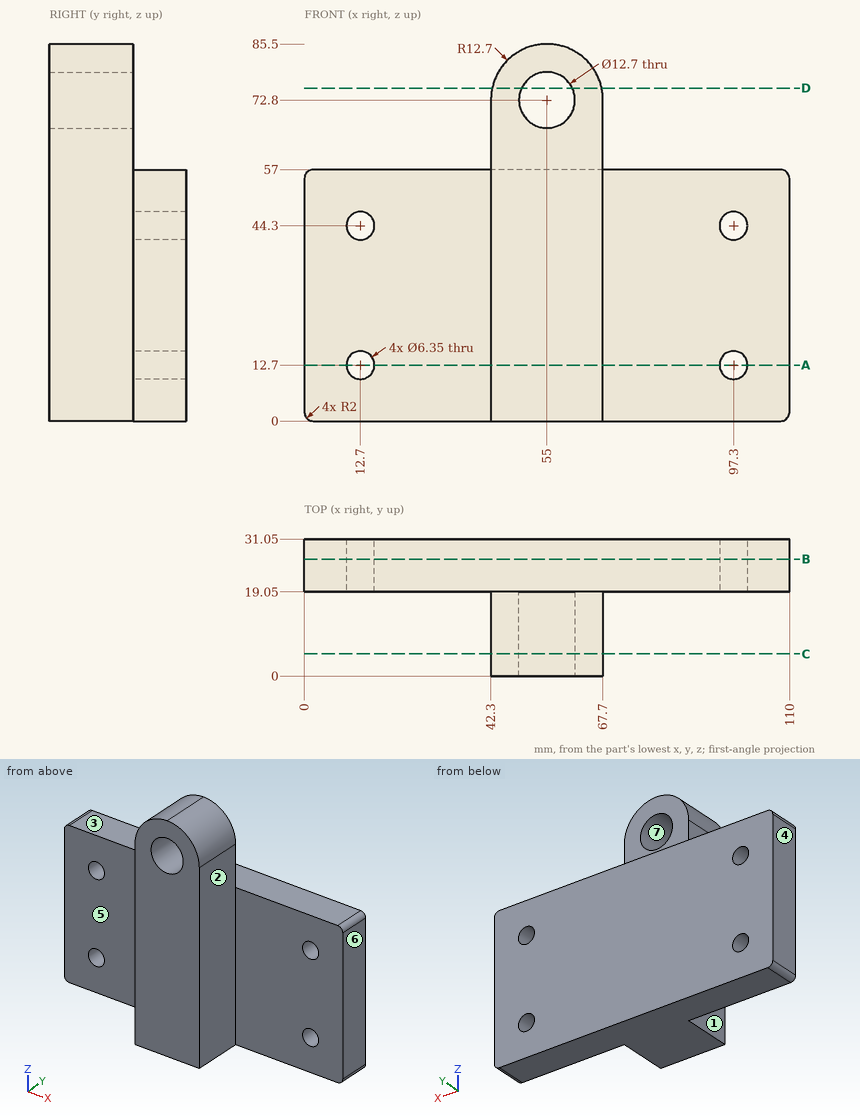
Design review of the part shown in the three views and the two pictorial views. Dimensions are in mm from the part's minimum x, y and z. A direction names the side the tool comes from. Round coordinates to 2 decimals unless told otherwise and drop trailing zeros. Write each loop counter-clockwise with the first axis right and the second up, starting at its lowest first coordinate (ties: lowest second). Pieces come first, ordered by that corner, then holes.
Item 1: Wall thickness on L1, parallel to X at y = 27, z = 44; L2, parallel to Z at x = 97, y = 22; L3, parallel to Z at x = 12, y = 26: over which ranges is each line inside the solid? List them lowest first.
Item 2: Consider section C-C on y = 5. Give the boundary of the cut face in (x, z), and give its area (3 significant figures).
Item 3: For the marked faces 1, 2, 3 and 4, list the 3-axis set-ups (+Z, -Z, +X, -X, +Y, -Y) from which the entire face can be reached by the end or side of a thin tool; tool diameter is ignored.
Item 4: Consider section B-B on y = 26.5. Give the boundary of the cut face in (x, z) (3 decimals), and give its area (3 significant figures).
Item 5: Draft analysis for pull direction X (two halves, no side actions). For the marked faces 5, 6 and 7, state which applies: released by +X, released by -X, zero draft, split by the parting line, or undercut.
Item 6: For pin 1 Ø9.5 at (x, y) = (73.5, 25) entering from +Z; pin 2 Ø15 at (y, z) = (10.5, 31) entering from -X; pin 3 Ø5 at (x, z) = (23.5, 34) entering from -Y, all flat-tipped, find the tip position at first contact; note any pin that passes through.
Item 7: Consider section D-D on z = 75.5. Give the boundary of the cut face in (x, y).
Item 8: Consider section A-A on z = 12.7. Give the boundary of the cut face in (x, y) (3 decimals), and give its area (3 significant figures).
Check values:
1. L1: x = 0 to 9.54, 15.86 to 94.14, 100.46 to 110
1. L2: z = 0 to 9.54, 15.86 to 41.14, 47.46 to 57
1. L3: z = 0 to 9.6, 15.8 to 41.2, 47.4 to 57
2. outline: (42.3, 0) - (67.7, 0) - (67.7, 72.8) arc R12.7 ccw to (42.3, 72.8) - close; hole circle Ø12.7 at (55, 72.8)
2. area: 1,980 mm2
3. face 1: +Z, -Z, -X, -Y
3. face 2: +Z, -Z, +X, -Y
3. face 3: +Z, +X, -X, +Y
3. face 4: +Z, -Z, -X, +Y, -Y
4. outline: (0, 2) arc R2 ccw to (2, 0) - (108, 0) arc R2 ccw to (110, 2) - (110, 55) arc R2 ccw to (108, 57) - (2, 57) arc R2 ccw to (0, 55) - close; hole circle Ø6.35 at (12.7, 12.7); hole circle Ø6.35 at (12.7, 44.3); hole circle Ø6.35 at (97.3, 12.7); hole circle Ø6.35 at (97.3, 44.3)
4. area: 6,140 mm2
5. face 5: zero draft
5. face 6: released by +X
5. face 7: undercut
6. pin 1: stops at z = 57
6. pin 2: stops at x = 42.3
6. pin 3: stops at y = 19.05
7. outline: (42.59, 0) - (49.25, 0) - (49.25, 19.05) - (42.59, 19.05) - close; (60.75, 0) - (67.41, 0) - (67.41, 19.05) - (60.75, 19.05) - close
8. outline: (0, 19.05) - (9.525, 19.05) - (9.525, 31.05) - (0, 31.05) - close; (15.875, 19.05) - (42.3, 19.05) - (42.3, 0) - (67.7, 0) - (67.7, 19.05) - (94.125, 19.05) - (94.125, 31.05) - (15.875, 31.05) - close; (100.475, 19.05) - (110, 19.05) - (110, 31.05) - (100.475, 31.05) - close
8. area: 1,650 mm2
